Verification items for the finished model (mm, model axes). A direction names the side the tool comes from. Coordinates: 2 decimals unless noted, no trailing zeros. Loops run counter-clockwise (first coordinate to the right, second up) from the corner with the lowest first, then second, coordinate; pieces in that order, holes last. Notation, with made-up numbers: (-7.5, 28.5) - (40.5, 28.5) arc R19 ccw to (40.5, 36.5) - close; hole circle Ø7 at (-18.5, 81.25). An arc over 180 degrees is marked (long way). One line per item, written item: value. Start each with the question number.
(1) Draft check along Y on faces 1 (the face through (3, 26, 0)), 2 (the face through (10, -5, 8)), 3 (the face through (10, 45.5, 7)), 4 (the face through (3.5, 20, 3)). Enter one of: +Y half, -Y half, draft (parallel to the pull), parting line (faces both ways), or undercut.
(2) Thickness scan on probe 1 along Y at (x, z) = (16, 4); probe 2 along X at (y, z) = (24, 9); probe 3 along X at (y, z) = (33, 10.5). Record the ranges inside material, lowest first. Write a range as [from, to].
(3) Section check C-C (y = 41.5). Record the boundary of the cut face in (x, z), plus the area to 3 significant figures.
(4) Gauge pin test, flat ends, axial feed: P1, Ø5.5, axis at y = 16, z = 12.5, coming from the +X side; P2, Ø1, axis at y = 37, z = 9.5, coming from the -X side; P3, Ø8, axis at x = 56.5, z = 13, coming from the -Y side. Record the tip position at first contact, or that the pin passes through.
(5) Section check A-A (x = 15). Record the boundary of the cut face in (y, z).
(6) Set-up check for faces 5 (the face through (-6, 21, 7)), 6 (the face through (3, 26, 15)), 7 (the face through (2.5, 20, 7)), 8 (the face through (-2.96, 19.49, 6.39)), 9 (the face through (12, 37, 3)): record each of +Z, -Z, +X, -X, +Y, -Y from which the full face is reachable in a straight line by a thin tool's end or side.
(7) Section check D-D (z = 14). Record the boundary of the cut face in (x, y).
(8) Section check B-B (z = 7.5). Record the boundary of the cut face in (x, y).
Autodesk Inventor part; units mm, degrees
ref_plane "Work Plane1" through (0, 0, 7.5) normal (0, 0, 1) x (1, 0, 0)
ref_plane "YZ Plane" through (0, 0, 0) normal (1, 0, 0) x (0, 1, 0)
ref_plane "XZ Plane" through (0, 0, 0) normal (0, 1, 0) x (-1, 0, 0)
sketch "Sketch1" plane through (0, 0, 0) normal (0, 0, 1) x (1, 0, 0)
  line L0 (0, 0) -> (20.25, 0)
  line L1 (20.25, 0) -> (20.25, 40.5)
  line L2 (20.25, 40.5) -> (0, 40.5)
  line L3 (0, 40.5) -> (0, 0)
  dimension "d0" = 40.5
  dimension "d1" = 20.25
extrude "Extrusion1" add sketch "Sketch1" along normal blind 15
sketch "Sketch2" plane through (0, 0, 15) normal (0, 0, 1) x (1, 0, 0)
  line L0 (3.5, 37) -> (20.25, 37)
  line L1 (20.25, 37) -> (20.25, 3.5)
  line L2 (20.25, 3.5) -> (3.5, 3.5)
  line L3 (3.5, 3.5) -> (3.5, 37)
  line L4 (20.25, 0) -> (20.25, 40.5)
  line L5 (20.25, 40.5) -> (0, 40.5)
  line L6 (0, 0) -> (20.25, 0)
  dimension "d4" = 16.75
  dimension "d5" = 3.5
  dimension "d6" = 3.5
extrude "Extrusion2" cut sketch "Sketch2" against normal blind 15
ref_plane "Work Plane1" through (0, 0, 7.5) normal (0, 0, 1) x (1, 0, 0)
sketch "Sketch3" plane through (0, 0, 7.5) normal (0, 0, 1) x (1, 0, 0)
  line L0 (2.5, 38) -> (20.25, 38)
  line L1 (20.25, 38) -> (20.25, 2.5)
  line L2 (20.25, 2.5) -> (2.5, 2.5)
  line L3 (2.5, 2.5) -> (2.5, 38)
  line L4 (20.25, 0) -> (20.25, 3.5)
  line L5 (20.25, 40.5) -> (0, 40.5)
  line L6 (0, 0) -> (20.25, 0)
  line L7 (0, 40.5) -> (0, 0)
  dimension "d10" = 2.5
  dimension "d11" = 2.5
  dimension "d12" = 2.5
extrude "Extrusion3" cut sketch "Sketch3" along normal mid plane 5
sketch "Sketch4" plane through (20.25, 40.5, 15) normal (1, 0, 0) x (0, 0, -1)
  line L0 (15, 0) -> (0, 0)
  line L1 (0, 0) -> (15, 0)
  line L2 (15, 0) -> (15, 5)
  line L3 (15, 5) -> (0, 5)
  line L4 (0, 5) -> (0, 0)
  line L5 (15, -40.5) -> (15, -37)
  line L6 (15, -40.5) -> (0, -40.5)
  line L7 (0, -40.5) -> (0, -45.5)
  line L8 (0, -45.5) -> (15, -45.5)
  line L9 (15, -45.5) -> (15, -40.5)
  dimension "d15" = 5
  dimension "d16" = 5
extrude "Extrusion4" add sketch "Sketch4" against normal blind 20.25
sketch "Sketch5" plane through (0, 0, 15) normal (0, 0, 1) x (1, 0, 0)
  point P0 (0, 0)
sketch "Sketch6" plane through (20.25, 37, 10) normal (1, 0, 0) x (0, 0, -1)
  circle A0 centre (2.5, 4.5) radius 2.5
  circle A1 centre (2.5, -38) radius 2.5
  line L0 (10, 0) -> (10, 8.5)
  line L1 (0, 1) -> (5, 1)
  line L2 (10, 8.5) -> (-5, 8.5)
  line L3 (5, -34.5) -> (0, -34.5)
  point P0 (10, -37)
  dimension "d19" = 7.5
  dimension "d20" = 0
  dimension "d21" = 3.5
  dimension "d22" = 7.5
  dimension "d23" = 3.5
  dimension "d24" = 5
extrude "Extrusion5" add sketch "Sketch6" along normal blind 50
sketch "Sketch7" plane through (0, 0, 15) normal (0, 0, 1) x (1, 0, 0)
  line L0 (0, -5) -> (0, 45.5)
  line L1 (2.5, 2.5) -> (2.5, 38)
  point P0 (0, 0)
  dimension "d27" = 2.5
sketch "Sketch8" plane through (0, -5, 0) normal (-1, 0, 0) x (0, 0, 1)
  circle A0 centre (7.5, 25.5) radius 1.5
  line L0 (15, 50.5) -> (0, 50.5)
  line L1 (0, 0) -> (15, 0)
  line L2 (15, 0) -> (15, 50.5)
  line L3 (0, 50.5) -> (0, 0)
  point P0 (0, 5)
  dimension "d28" = 50.5
  dimension "d29" = 25
  dimension "d30" = 3
  dimension "d31" = 15
  dimension "d32" = 7.5
extrude "Extrusion6" add sketch "Sketch8" along normal blind 6 contours A0
properties part number "standlower"
Responses:
1. face 1: draft
1. face 2: -Y half
1. face 3: +Y half
1. face 4: undercut
2. probe 1: y = [-5, 3.5], [37, 45.5]
2. probe 2: x = [0, 2.5]
2. probe 3: x = [0, 3.5]
3. outline: (0, 0) - (20.25, 0) - (20.25, 5) - (70.25, 5) - (70.25, 10) - (20.25, 10) - (20.25, 15) - (0, 15) - close
3. area: 554 mm²
4. P1: stops at x = 3.5
4. P2: stops at x = 0
4. P3: stops at y = -3
5. outline: (-5, 0) - (3.5, 0) - (3.5, 5) - (2.5, 5) - (2.5, 10) - (3.5, 10) - (3.5, 15) - (-5, 15) - close; (37, 0) - (45.5, 0) - (45.5, 15) - (37, 15) - (37, 10) - (38, 10) - (38, 5) - (37, 5) - close
6. face 5: +Z, -Z, -X, +Y, -Y
6. face 6: +Z, +X, -X, +Y, -Y
6. face 7: +X
6. face 8: -X
6. face 9: +Z, -Z, +X
7. outline: (0, -5) - (20.25, -5) - (20.25, 3.5) - (3.5, 3.5) - (3.5, 37) - (20.25, 37) - (20.25, 45.5) - (0, 45.5) - close
8. outline: (-6, 19) - (0, 19) - (0, -5) - (20.25, -5) - (20.25, -3.5) - (70.25, -3.5) - (70.25, 1.5) - (20.25, 1.5) - (20.25, 2.5) - (2.5, 2.5) - (2.5, 38) - (20.25, 38) - (20.25, 39) - (70.25, 39) - (70.25, 44) - (20.25, 44) - (20.25, 45.5) - (0, 45.5) - (0, 22) - (-6, 22) - close
